Verification items for the finished model (mm, model axes). A direction names the side the tool comes from. Coordinates: 2 decimals unless noted, no trailing zeros. Order: outer loops, then holes, each group sorted by start corner. A loop starts at its lowest first (then second) coordinate and runs counter-clockwise, first axis right, second up. Notation, with made-up numbers: (38.25, 9) - (65.25, 9) arc R21 cw to (65.25, 35) - close; hole circle Ø4 at (-27.75, -26.5). An arc over 180 degrees is marked (long way). Answer as CSV lines item,"result". Start each with the question number.
1. Go/stop test with a flat-tipped pin: pin 1 (4 mm diameter, centred on x = -34.5, y = 31.5, fed in from +Z). Record where the tip stops, or that it passes through.
2. Mould release check, pull along Y, two halves, no side actions. Record for faces 5 (the flat face through (-15, -89.5, 3)), 6 (the flat face through (-60, 69.5, 11)), 7 (the flat face through (62, -1, 3)): pulls with the +Y half, pulls with the -Y half, needs draft (parallel to the pull), parting line crosses it, or undercut.
3. Section check D-D (x = 19.5). Record the cut outline in (y, z).
4. Material ranges on L1, parallel to Y at x = -42.5, z = 12; L2, parallel to X at y = 82.5, z = 8.5; L3, parallel to Z at x = -23.5, y = -6, recorded low to high. Write a range as [from, to].
5. Section check B-B (x = 50). Record the cut outline in (y, z), and give its area (3 significant figures).
6. Set-up check for faces 1 (the flat face through (15, 89.5, 3)), 2 (the flat face through (-58.5, 78, 11)), 3 (the flat face through (60, 69.5, 11)), 4 (the flat face through (-42, 88, 11)): record each of +Z, -Z, +X, -X, +Y, -Y from which the full face is reachable in a straight line by a thin tool's end or side.
7. Section check C-C (y = -73.5). Record the cut outline in (x, z), and give its area (3 significant figures).
8. Section check A-A (z = 7). Record the cut outline in (x, y).
from build123d import *

# Parameters (mm, degrees)
SKETCH_1_W      = 124
SKETCH_1_H      = 179
EXTRUDE_1_DEPTH = 4
EXTRUDE_2_DEPTH = 15


with BuildPart() as part:
    # 草圖1 → 填料-伸長1 (new body)
    with BuildSketch(Plane.XY):
        Rectangle(SKETCH_1_W, SKETCH_1_H)
    extrude(amount=EXTRUDE_1_DEPTH)

    # 草圖3 → 填料-伸長2 (add)
    with BuildSketch(Plane.XY.offset(4)):
        Polygon((-62, 89.5), (-62, 69.5), (-58.5, 69.5), (-58.5, 86), (-42, 86), (-42, 89.5), align=None)
        Polygon((42, 86), (42, 89.5), (62, 89.5), (62, 69.5), (58.5, 69.5), (58.5, 86), align=None)
        Polygon((62, -89.5), (62, -69.5), (58.5, -69.5), (58.5, -86), (42, -86), (42, -89.5), align=None)
        Polygon((-42, -86), (-42, -89.5), (-62, -89.5), (-62, -69.5), (-58.5, -69.5), (-58.5, -86), align=None)
    extrude(amount=EXTRUDE_2_DEPTH)


solid = part.part
Evaluation:
1,pin 1,"stops at z = 4"
2,face 5,"pulls with the -Y half"
2,face 6,"undercut"
2,face 7,"needs draft"
3,outline,"(-89.5, 0) - (89.5, 0) - (89.5, 4) - (-89.5, 4) - close"
4,L1,"y = [-89.5, -86], [86, 89.5]"
4,L2,"x = [-62, -58.5], [58.5, 62]"
4,L3,"z = [0, 4]"
5,outline,"(-89.5, 0) - (89.5, 0) - (89.5, 19) - (86, 19) - (86, 4) - (-86, 4) - (-86, 19) - (-89.5, 19) - close"
5,area,"821 mm²"
6,face 1,"+Z, -Z, +X, -X, +Y"
6,face 2,"+Z"
6,face 3,"+Z, +X, -X"
6,face 4,"+Z, +Y, -Y"
7,outline,"(-62, 0) - (62, 0) - (62, 19) - (58.5, 19) - (58.5, 4) - (-58.5, 4) - (-58.5, 19) - (-62, 19) - close"
7,area,"601 mm²"
8,outline,"(-62, -89.5) - (-42, -89.5) - (-42, -86) - (-58.5, -86) - (-58.5, -69.5) - (-62, -69.5) - close; (-62, 69.5) - (-58.5, 69.5) - (-58.5, 86) - (-42, 86) - (-42, 89.5) - (-62, 89.5) - close; (42, -89.5) - (62, -89.5) - (62, -69.5) - (58.5, -69.5) - (58.5, -86) - (42, -86) - close; (42, 86) - (58.5, 86) - (58.5, 69.5) - (62, 69.5) - (62, 89.5) - (42, 89.5) - close"
